from build123d import *

# Parameters (mm, degrees)
ESBO_O1_W                     = 4.75
ESBO_O1_H                     = 15
RESSALTO_EXTRUS_O1_DEPTH      = 4.4
ESBO_O2_R                     = 1.15
RESSALTO_EXTRUS_O2_DEPTH      = 1.5
RESSALTO_EXTRUS_O2_DEPTH_BACK = 18
ESBO_O3_R                     = 3.5
RESSALTO_EXTRUS_O3_DEPTH      = 1
ESBO_O4_R                     = 1.15
ESBO_O4_R_2                   = 0.5
CORTE_EXTRUS_O1_DEPTH         = 0.7
ESBO_O5_W                     = 1.5
ESBO_O5_H                     = 14
CORTE_EXTRUS_O2_DEPTH         = 1.3


with BuildPart() as part:
    # Esboço1 → Ressalto-extrusão1 (new body)
    with BuildSketch(Plane.XY):
        Rectangle(ESBO_O1_W, ESBO_O1_H)
    extrude(amount=RESSALTO_EXTRUS_O1_DEPTH)

    # Esboço2 → Ressalto-extrusão2 (add, two sides)
    with BuildSketch(Plane.XZ.offset(7.5)) as ressalto_extrus_o2_sk:
        with Locations((0, 3)):
            Circle(ESBO_O2_R)
    extrude(amount=RESSALTO_EXTRUS_O2_DEPTH)
    extrude(ressalto_extrus_o2_sk.sketch, amount=-RESSALTO_EXTRUS_O2_DEPTH_BACK)

    # Esboço3 → Ressalto-extrusão3 (add)
    with BuildSketch(Plane(origin=(0, 8.9, 0), x_dir=(1, 0, 0), z_dir=(0, 1, 0))):
        with Locations((0, -3)):
            Circle(ESBO_O3_R)
    extrude(amount=-RESSALTO_EXTRUS_O3_DEPTH)

    # Esboço4 → Corte-extrusão1 (cut)
    with BuildSketch(Plane(origin=(0, 10.5, 0), x_dir=(1, 0, 0), z_dir=(0, 1, 0))):
        with Locations((0, -3)):
            Circle(ESBO_O4_R)
        with Locations((0, -3)):
            Circle(ESBO_O4_R_2, mode=Mode.SUBTRACT)
    extrude(amount=-CORTE_EXTRUS_O1_DEPTH, mode=Mode.SUBTRACT)

    # Esboço5 → Corte-extrusão2 (cut)
    with BuildSketch(Plane.XY.offset(4.4)):
        Rectangle(ESBO_O5_W, ESBO_O5_H)
    extrude(amount=-CORTE_EXTRUS_O2_DEPTH, mode=Mode.SUBTRACT)


solid = part.part
Source: CAD feature listing. Evaluate the final solid. Frame: model axes, mm. A direction names the side the tool comes from. Give positions to 0.01 mm unless a question says otherwise; leave off trailing zeros. Write each loop counter-clockwise with the first axis right and the second up, starting at its lowest first coordinate (ties: lowest second). Pieces come first, ordered by that corner, then holes. Notation, with made-up numbers: (71.5, 19.25) -> (77.5, 19.25) arc R20 cw to (77.5, 25.25) -> close; hole circle Ø2 at (-32.75, 61.25). An arc over 180 degrees is marked (long way). Return JSON: item names as keys, results as strings. Group by question number.
1. Pin query (flat end, axial travel): pin 1 Ø1 at (x, z) = (-1, 1.5) entering from +Y; pin 2 Ø1.2 at (x, y) = (-0.5, 1) entering from +Z; pin 3 Ø3.5 at (x, z) = (-1, 1.5) entering from -Y; pin 4 Ø1 at (y, z) = (-5, 2.5) entering from +X (3 decimals). Return the tip coordinate at first contact, or that it passes through.
2. Section D-D, the plane x = -1.5. Output: boundary loops of the cut face in (y, z).
3. Access query for faces 1 (the face through (-0.75, 0, 4)), 2 (the face through (-0.249, -8.24, 1.877)), 3 (the face through (-2.375, 0, 2)), 4 (the face through (-0.065, 10.155, 2.504)). Directions: +Z, -Z, +X, -X, +Y, -Y. A direction counts if a zero-diameter tool reaches every point of the face in a straight line with its end or side. Return the directions, or none.
4. Material intervals for line 1 (Y direction, x = 1, z = 0.75); line 2 (X direction, y = -5.75, z = 1.5) (3 decimals); line 3 (Z direction, x = 0, y = 4.5), sorted ascending. Write a range as from..to.
5. Section B-B, the plane y = 0.5. Output: boundary loops of the cut face in (x, z) (3 decimals).
6. Section C-C, the plane x = 0. Output: boundary loops of the cut face in (y, z), then the cut area to 3 significant figures.
7. Mould query, pull axis X, two halves, no side actions, for faces 5 (the face through (0.75, 0, 4)), 6 (the face through (-0.249, 9.344, 1.877)), 7 (the face through (0, 10.5, 3)). Classes: +X half, -X half, draft (parallel to the pull), parting line (faces both ways), or undercut.
8. Section A-A, the plane x = 2. Output: boundary loops of the cut face in (y, z).
Determined:
{
 "1": {"pin 1": "stops at y = 8.9", "pin 2": "stops at z = 4.4", "pin 3": "stops at y = -9", "pin 4": "stops at x = 2.375"},
 "2": {"outline": "(-7.5, 0) -> (7.5, 0) -> (7.5, 4.4) -> (-7.5, 4.4) -> close; (7.9, -0.16) -> (8.9, -0.16) -> (8.9, 6.16) -> (7.9, 6.16) -> close"},
 "3": {"face 1": "+Z", "face 2": "-Y", "face 3": "+Z, -Z, -X, -Y", "face 4": "+Y"},
 "4": {"line 1": "y = -7.5..7.5, 7.9..8.9", "line 2": "x = -2.375..2.375", "line 3": "z = 0..3.1"},
 "5": {"outline": "(-2.375, 0) -> (2.375, 0) -> (2.375, 4.4) -> (0.75, 4.4) -> (0.75, 3.1) -> (-0.75, 3.1) -> (-0.75, 4.4) -> (-2.375, 4.4) -> close"},
 "6": {"outline": "(-9, 1.85) -> (-7.5, 1.85) -> (-7.5, 0) -> (7.5, 0) -> (7.5, 1.85) -> (7.9, 1.85) -> (7.9, -0.5) -> (8.9, -0.5) -> (8.9, 1.85) -> (9.8, 1.85) -> (9.8, 2.5) -> (10.5, 2.5) -> (10.5, 3.5) -> (9.8, 3.5) -> (9.8, 4.15) -> (8.9, 4.15) -> (8.9, 6.5) -> (7.9, 6.5) -> (7.9, 4.15) -> (7.5, 4.15) -> (7.5, 4.4) -> (7, 4.4) -> (7, 3.1) -> (-7, 3.1) -> (-7, 4.4) -> (-7.5, 4.4) -> (-7.5, 4.15) -> (-9, 4.15) -> close", "area": "61.9 mm2"},
 "7": {"face 5": "undercut", "face 6": "parting line", "face 7": "draft"},
 "8": {"outline": "(-7.5, 0) -> (7.5, 0) -> (7.5, 4.4) -> (-7.5, 4.4) -> close; (7.9, 0.13) -> (8.9, 0.13) -> (8.9, 5.87) -> (7.9, 5.87) -> close"}
}
